Input: part model. Units: mm. Frame: model coordinates. A direction names the side the tool comes from. Round coordinates to 2 decimals unless told otherwise and drop trailing zeros. Loops run counter-clockwise (first coordinate to the right, second up) from the corner with the lowest first, then second, coordinate; pieces in that order, holes last. Notation, with made-up numbers: (8, 29.5) -> (16, 29.5) arc R18 cw to (16, 36.5) -> close; hole circle Ø2 at (-1, -32). An arc over 180 degrees is marked (long way). Answer in a Markdown table with one row per item. Add a question column.
Q1. Section D-D, the plane y = 3. Output: boundary loops of the cut face in (x, z).
Q2. Section A-A, the plane z = 8.5. Output: boundary loops of the cut face in (x, y) (1 decimal), and give its area (3 significant figures).
Q3. Pin query (flat end, axial travel): pin 1 (2 mm diameter, centred on y = 51.5, z = 6.5, fed in from -X); pin 2 (6 mm diameter, centred on x = -13, z = 3.5, fed in from -Y); pin 3 (1.5 mm diameter, centred on x = 10.5, y = -14, fed in from +Z). Return the tip coordinate at first contact, or that it passes through.
Q4. Section C-C, the plane x = -36.5. Output: boundary loops of the cut face in (y, z), and give its area (3 significant figures).
Q5. Mould query, pull axis Y, two halves, no side actions, for faces 1 (the face through (0.1, 66.4, 5.1)), 2 (the face through (0.1, 67.2, 4.1)), 3 (the face through (-25.1, -28.3, 4.1)). Classes: pulls with the +Y half, pulls with the -Y half, needs draft (parallel to the pull), parting line crosses it, or undercut.
Q6. Reachability of faces 4 (the face through (11.18, 34.55, 5.07)), 5 (the face through (-11.96, 35.89, 4.08)), 6 (the face through (24.38, -27.9, 4.08)) from +Z, -Z, +X, -X, +Y, -Y: full face, straight path, thin tool, end or side. Return the list, or none.
Q7. Section B-B, the plane y = -21.5. Output: boundary loops of the cut face in (x, z).
Q8. Ray query, L1, parallel to X at y = -21, z = 4.5; L2, parallel to X at y = -30, z = 4.5; L3, parallel to Z at x = -3, y = 55.5. Return the intervals inside material, ascending. Write a range as from..to.
```python
from build123d import *

# Parameters (mm, degrees)
F1_DEPTH = 10
F3_DEPTH = 10
F0_R     = 7.5
F4_DEPTH = 2


with BuildPart() as f1:
    # F0 (on Top) → F1 (new body)
    with BuildSketch(Plane.XY):
        with BuildLine():
            ThreePointArc((60.856366, -24.384369), (36.710284, -7.376819), (10.3731, 5.988912))
            ThreePointArc((10.3731, 5.988912), (11.966629, 35.480448), (9.3107, 64.895344))
            ThreePointArc((9.3107, 64.895344), (0, 67.2), (-9.3107, 64.895344))
            ThreePointArc((-9.3107, 64.895344), (-11.966629, 35.480448), (-10.3731, 5.988912))
            ThreePointArc((-10.3731, 5.988912), (-36.710284, -7.376819), (-60.856366, -24.384369))
            ThreePointArc((-60.856366, -24.384369), (-58.196907, -33.6), (-51.545666, -40.510974))
            ThreePointArc((-51.545666, -40.510974), (-24.743655, -28.103629), (0, -11.977824))
            ThreePointArc((0, -11.977824), (24.743655, -28.103629), (51.545666, -40.510974))
            ThreePointArc((51.545666, -40.510974), (58.196907, -33.6), (60.856366, -24.384369))
        make_face()
        with BuildLine():
            ThreePointArc((-7.5, 63.559028), (0, 65.2), (7.5, 63.559028))
            ThreePointArc((7.5, 63.559028), (9.985947, 34.169463), (8.191847, 4.729565))
            ThreePointArc((8.191847, 4.729565), (34.584597, -8.436648), (58.793733, -25.284323))
            ThreePointArc((58.793733, -25.284323), (56.464856, -32.6), (51.293733, -38.274704))
            ThreePointArc((51.293733, -38.274704), (24.59865, -25.732816), (0, -9.45913))
            ThreePointArc((0, -9.45913), (-24.59865, -25.732816), (-51.293733, -38.274704))
            ThreePointArc((-51.293733, -38.274704), (-56.464856, -32.6), (-58.793733, -25.284323))
            ThreePointArc((-58.793733, -25.284323), (-34.584597, -8.436648), (-8.191847, 4.729565))
            ThreePointArc((-8.191847, 4.729565), (-9.985947, 34.169463), (-7.5, 63.559028))
        make_face(mode=Mode.SUBTRACT)
    extrude(amount=F1_DEPTH)

    # F2 (on face) → F3 (cut)
    with BuildSketch(Plane.XY.offset(10)):
        with BuildLine():
            ThreePointArc((-8.585798, 64.368588), (-11.175251, 34.960479), (-9.502098, 5.486039))
            ThreePointArc((-9.502098, 5.486039), (-35.864289, -7.802188), (-60.037731, -24.748774))
            ThreePointArc((-60.037731, -24.748774), (-57.504087, -33.2), (-51.451933, -39.619813))
            ThreePointArc((-51.451933, -39.619813), (-24.689038, -27.158291), (0, -10.972078))
            ThreePointArc((0, -10.972078), (24.689038, -27.158291), (51.451933, -39.619813))
            ThreePointArc((51.451933, -39.619813), (57.504087, -33.2), (60.037731, -24.748774))
            ThreePointArc((60.037731, -24.748774), (35.864289, -7.802188), (9.502098, 5.486039))
            ThreePointArc((9.502098, 5.486039), (11.175251, 34.960479), (8.585798, 64.368588))
            ThreePointArc((8.585798, 64.368588), (0, 66.4), (-8.585798, 64.368588))
        make_face()
        with BuildLine():
            ThreePointArc((7.5, 63.559028), (9.985947, 34.169463), (8.191847, 4.729565))
            ThreePointArc((8.191847, 4.729565), (34.584597, -8.436648), (58.793733, -25.284323))
            ThreePointArc((58.793733, -25.284323), (56.464856, -32.6), (51.293733, -38.274704))
            ThreePointArc((51.293733, -38.274704), (24.59865, -25.732816), (0, -9.45913))
            ThreePointArc((0, -9.45913), (-24.59865, -25.732816), (-51.293733, -38.274704))
            ThreePointArc((-51.293733, -38.274704), (-56.464856, -32.6), (-58.793733, -25.284323))
            ThreePointArc((-58.793733, -25.284323), (-34.584597, -8.436648), (-8.191847, 4.729565))
            ThreePointArc((-8.191847, 4.729565), (-9.985947, 34.169463), (-7.5, 63.559028))
            ThreePointArc((-7.5, 63.559028), (0, 65.2), (7.5, 63.559028))
        make_face(mode=Mode.SUBTRACT)
    extrude(amount=-F3_DEPTH, mode=Mode.SUBTRACT)

    # F0 (on Top) → F4 (join)
    with BuildSketch(Plane.XY):
        with BuildLine():
            ThreePointArc((60.856366, -24.384369), (36.710284, -7.376819), (10.3731, 5.988912))
            ThreePointArc((10.3731, 5.988912), (11.966629, 35.480448), (9.3107, 64.895344))
            ThreePointArc((9.3107, 64.895344), (0, 67.2), (-9.3107, 64.895344))
            ThreePointArc((-9.3107, 64.895344), (-11.966629, 35.480448), (-10.3731, 5.988912))
            ThreePointArc((-10.3731, 5.988912), (-36.710284, -7.376819), (-60.856366, -24.384369))
            ThreePointArc((-60.856366, -24.384369), (-58.196907, -33.6), (-51.545666, -40.510974))
            ThreePointArc((-51.545666, -40.510974), (-24.743655, -28.103629), (0, -11.977824))
            ThreePointArc((0, -11.977824), (24.743655, -28.103629), (51.545666, -40.510974))
            ThreePointArc((51.545666, -40.510974), (58.196907, -33.6), (60.856366, -24.384369))
        make_face()
        with BuildLine():
            ThreePointArc((-7.5, 63.559028), (0, 65.2), (7.5, 63.559028))
            ThreePointArc((7.5, 63.559028), (9.985947, 34.169463), (8.191847, 4.729565))
            ThreePointArc((8.191847, 4.729565), (34.584597, -8.436648), (58.793733, -25.284323))
            ThreePointArc((58.793733, -25.284323), (56.464856, -32.6), (51.293733, -38.274704))
            ThreePointArc((51.293733, -38.274704), (24.59865, -25.732816), (0, -9.45913))
            ThreePointArc((0, -9.45913), (-24.59865, -25.732816), (-51.293733, -38.274704))
            ThreePointArc((-51.293733, -38.274704), (-56.464856, -32.6), (-58.793733, -25.284323))
            ThreePointArc((-58.793733, -25.284323), (-34.584597, -8.436648), (-8.191847, 4.729565))
            ThreePointArc((-8.191847, 4.729565), (-9.985947, 34.169463), (-7.5, 63.559028))
        make_face(mode=Mode.SUBTRACT)
        with BuildLine():
            ThreePointArc((8.191847, 4.729565), (9.985947, 34.169463), (7.5, 63.559028))
            ThreePointArc((7.5, 63.559028), (0, 65.2), (-7.5, 63.559028))
            ThreePointArc((-7.5, 63.559028), (-9.985947, 34.169463), (-8.191847, 4.729565))
            ThreePointArc((-8.191847, 4.729565), (-34.584597, -8.436648), (-58.793733, -25.284323))
            ThreePointArc((-58.793733, -25.284323), (-56.464856, -32.6), (-51.293733, -38.274704))
            ThreePointArc((-51.293733, -38.274704), (-24.59865, -25.732816), (0, -9.45913))
            ThreePointArc((0, -9.45913), (24.59865, -25.732816), (51.293733, -38.274704))
            ThreePointArc((51.293733, -38.274704), (56.464856, -32.6), (58.793733, -25.284323))
            ThreePointArc((58.793733, -25.284323), (34.584597, -8.436648), (8.191847, 4.729565))
        make_face()
        Circle(F0_R, mode=Mode.SUBTRACT)
        Circle(F0_R)
    extrude(amount=-F4_DEPTH)


solid = f1.part
```
Answer block:
| question | item | result |
|---|---|---|
| 1 | outline | (-17.15, -2) -> (17.15, -2) -> (17.15, 10) -> (15.22, 10) -> (15.22, 0) -> (-15.22, 0) -> (-15.22, 10) -> (-17.15, 10) -> close |
| 2 | outline | (-60.9, -24.4) arc R20 ccw to (-51.5, -40.5) arc R205.2 ccw to (0, -12) arc R205.2 ccw to (51.5, -40.5) arc R20 ccw to (60.9, -24.4) arc R205.2 ccw to (10.4, 6) arc R205.2 ccw to (9.3, 64.9) arc R20 ccw to (-9.3, 64.9) arc R205.2 ccw to (-10.4, 6) arc R205.2 ccw to start; hole (-60, -24.7) arc R19.2 ccw to (-51.5, -39.6) arc R204.4 ccw to (0, -11) arc R204.4 ccw to (51.5, -39.6) arc R19.2 ccw to (60, -24.7) arc R204.4 ccw to (9.5, 5.5) arc R204.4 ccw to (8.6, 64.4) arc R19.2 ccw to (-8.6, 64.4) arc R204.4 ccw to (-9.5, 5.5) arc R204.4 ccw to start |
| 2 | area | 328 mm^2 |
| 3 | pin 1 | x = -11.14 |
| 3 | pin 2 | y = -22.98 |
| 3 | pin 3 | z = 0 |
| 4 | outline | (-34.13, -2) -> (-7.25, -2) -> (-7.25, 10) -> (-8.18, 10) -> (-8.18, 0) -> (-33.24, 0) -> (-33.24, 10) -> (-34.13, 10) -> close |
| 4 | area | 71.9 mm^2 |
| 5 | face 1 | undercut |
| 5 | face 2 | pulls with the +Y half |
| 5 | face 3 | pulls with the -Y half |
| 6 | face 4 | +Z |
| 6 | face 5 | +Z, -Z, -X |
| 6 | face 6 | +Z, -Z, -Y |
| 7 | outline | (-57.25, -2) -> (-13.65, -2) -> (-13.65, 10) -> (-15.15, 10) -> (-15.15, 0) -> (-55.94, 0) -> (-55.94, 10) -> (-57.25, 10) -> close; (13.65, -2) -> (57.25, -2) -> (57.25, 10) -> (55.94, 10) -> (55.94, 0) -> (15.15, 0) -> (15.15, 10) -> (13.65, 10) -> close |
| 8 | L1 | -56.61..-55.3, -14.36..-12.87, 12.87..14.36, 55.3..56.61 |
| 8 | L2 | -59.82..-58.98, -29.97..-28.25, 28.25..29.97, 58.98..59.82 |
| 8 | L3 | -2..0 |
